Verification items for the finished model (mm, model axes). A direction names the side the tool comes from. Coordinates: 2 decimals unless noted, no trailing zeros. Write each loop counter-clockwise with the first axis right and the second up, starting at its lowest first coordinate (ties: lowest second). Pieces come first, ordered by that corner, then holes. Notation, with made-up numbers: (23, -25.5) - (44, -25.5) arc R11 cw to (44, -11.5) - close; hole circle Ø2 at (9.25, 41). An arc over 180 degrees is marked (long way). Use CSV: the item, a comma, the result in double quotes. Start each with the question number.
Autodesk Inventor part; units mm, degrees
ref_plane "YZ Plane" through (0, 0, 0) normal (1, 0, 0) x (0, 1, 0)
ref_plane "XZ Plane" through (0, 0, 0) normal (0, 1, 0) x (-1, 0, 0)
ref_plane "XY Plane" through (0, 0, 0) normal (0, 0, 1) x (1, 0, 0)
sketch "Sketch1" plane through (0, 0, 0) normal (0, 1, 0) x (-1, 0, 0)
  line L0 (16.5, 8) -> (-16.5, 8)
  line L1 (-16.5, 8) -> (-16.5, -8)
  line L2 (-16.5, -8) -> (16.5, -8)
  line L3 (16.5, -8) -> (16.5, 8)
  line L4 (16.5, 8) -> (-16.5, -8) construction
  line L5 (-16.5, 8) -> (16.5, -8) construction
  point P0 (0, 0)
  dimension "d0" = 16
  dimension "d1" = 33
extrude "Extrusion1" add sketch "Sketch1" along normal blind 2
sketch "Sketch2" plane through (0, 2, 0) normal (0, 1, 0) x (1, 0, 0)
  line L0 (-16.5, -8) -> (16.5, -8)
  line L1 (16.5, -8) -> (16.5, 8)
  line L2 (16.5, 8) -> (-16.5, 8)
  line L3 (-16.5, 8) -> (-16.5, -8)
  line L4 (16.5, -8) -> (9.5, -8)
  line L5 (9.5, -8) -> (9.5, 8)
  line L6 (9.5, 8) -> (16.5, 8)
  line L7 (16.5, 8) -> (16.5, -8)
  point P0 (0, 0)
  dimension "d4" = 7
extrude "Extrusion2" add sketch "Sketch2" along normal blind 20 contours L5 L2 L1 L0
sketch "Sketch3" plane through (16.5, 0, 8) normal (1, 0, 0) x (0, 0, -1)
  line L0 (0, 0) -> (16, 0)
  line L1 (16, 0) -> (16, 22)
  line L2 (0, 22) -> (16, 22)
  line L3 (0, 0) -> (0, 22)
  line L4 (10.75, 18) -> (5.25, 18)
  line L5 (5.25, 18) -> (5.25, 2)
  line L6 (5.25, 2) -> (10.75, 2)
  line L7 (10.75, 2) -> (10.75, 18)
  line L8 (10.75, 18) -> (5.25, 2) construction
  line L9 (5.25, 18) -> (10.75, 2) construction
  circle A0 centre (8, 18) radius 4
  line L10 (0, 22) -> (16, 22)
  line L11 (4, 18) -> (12, 18)
  line L12 (12, 18) -> (12, 22)
  line L13 (12, 22) -> (4, 22)
  line L14 (4, 22) -> (4, 18)
  point P0 (8, 0)
  point P1 (8, 10)
  dimension "d11" = 8
  dimension "d7" = 4
  dimension "d8" = 16
  dimension "d9" = 5.5
  dimension "d10" = 8
extrude "Extrusion3" cut sketch "Sketch3" against normal blind 4 contours A0 L7 L6 L5 | L5 L4 L7 A0
extrude "Extrusion4" cut sketch "Sketch3" against normal blind 5 contours L2 A0 L14 | L12 A0 L2 | A0 L11 L4 | L11 L5 A0 | A0 L7 L11 | L5 L4 L7 A0
sketch "Sketch4" plane through (16.5, 0, 8) normal (1, 0, 0) x (0, 0, -1)
  line L0 (5.25, 2) -> (5.25, 15.0953)
  line L1 (10.75, 15.0953) -> (10.75, 2)
  line L2 (5.25, 14) -> (10.75, 14)
  line L3 (10.75, 14) -> (10.75, 7.5)
  line L4 (10.75, 7.5) -> (5.25, 7.5)
  line L5 (5.25, 7.5) -> (5.25, 14)
  line L6 (10.75, 2) -> (5.25, 2)
  point P0 (8, 0)
  dimension "d16" = 5.5
  dimension "d17" = 6.5
extrude "Extrusion5" add sketch "Sketch4" against normal blind 2 contours L0 L2 L1 L4
fillet "Fillet1" radius 2.75 2 edges at (15.5, 7.5, -2.75) (15.5, 7.5, 2.75)
properties part number "leg_hind_upper_joint"
Q1. Cross-section at A-A (y = 9.25). Record the cut outline in (x, z), plus the area to 3 significant figures.
Q2. Cross-section at C-C (y = 2.75). Record the cut outline in (x, z).
Q3. Tool access check on faces 1 (the flat face through (12.5, 9, 0)), 2 (the cylindrical face through (15.49, 6.72, -1.92)), 3 (the flat face through (14, 20, -4)), 4 (the flat face through (-3, 2, 0)). Record the directions out of +Z, -Z, +X, -X, +Y, -Y that give a thin tool (end or side, any length) a straight path to the whole face; none if there is none.
Q4. Scan lines: line 1 along Z through (x, y) = (13, 7.25); line 2 along X through (y, z) = (13, 1.5); line 3 along Y through (x, z) = (-12, 4.25). Record each from-to range of solid material in increasing order. Write a range as from..to.
Q5. Gauge pin test, flat ends, axial feed: pin 1 (3 mm diameter, centred on x = -9, z = 1.5, fed in from -Y); pin 2 (6 mm diameter, centred on y = 8, z = -1.5, fed in from -X); pin 3 (8 mm diameter, centred on x = 5, y = 7.5, fed in from -Z); pin 4 (2 mm diameter, centred on x = -4.5, z = -5.5, fed in from +Y). Record the tip position at first contact, or that the pin passes through.
Q6. Cross-section at D-D (x = -4.5). Record the cut outline in (y, z).
Q7. Cross-section at B-B (z = -0.5). Record the cut outline in (x, y).
Q8. Release check for a two-part mould opening along Z. For faces 5 (the flat face through (16.5, 11, 0)), 6 (the flat face through (14, 9, 2.75)), 7 (the flat face through (10, 8, 8)), 8 (the flat face through (14, 8, -2.75)) record: released by +Z, released by -Z, zero draft, split by the parting line, or undercut.
Reply:
1,outline,"(9.5, -8) - (16.5, -8) - (16.5, 8) - (9.5, 8) - close; hole (12.5, -2.75) - (14.5, -2.75) - (14.5, 2.75) - (12.5, 2.75) - close"
1,area,"101 mm^2"
2,outline,"(9.5, -8) - (16.5, -8) - (16.5, -2.75) - (12.5, -2.75) - (12.5, 2.75) - (16.5, 2.75) - (16.5, 8) - (9.5, 8) - close"
3,face 1,"+Y"
3,face 2,"+X"
3,face 3,"+X, +Y"
3,face 4,"+Z, -Z, -X, +Y"
4,line 1,"-8..-2.75, 2.75..8"
4,line 2,"9.5..12.5, 14.5..16.5"
4,line 3,"0..2"
5,pin 1,"y = 0"
5,pin 2,"x = 9.5"
5,pin 3,"through"
5,pin 4,"y = 2"
6,outline,"(0, -8) - (2, -8) - (2, 8) - (0, 8) - close"
7,outline,"(-16.5, 0) - (16.5, 0) - (16.5, 2) - (12.5, 2) - (12.5, 14.03) - (11.5, 14.03) - (11.5, 22) - (9.5, 22) - (9.5, 2) - (-16.5, 2) - close; (14.5, 7.45) - (16.5, 7.45) - (16.5, 14) - (14.5, 14) - close"
8,face 5,"zero draft"
8,face 6,"undercut"
8,face 7,"released by +Z"
8,face 8,"undercut"
